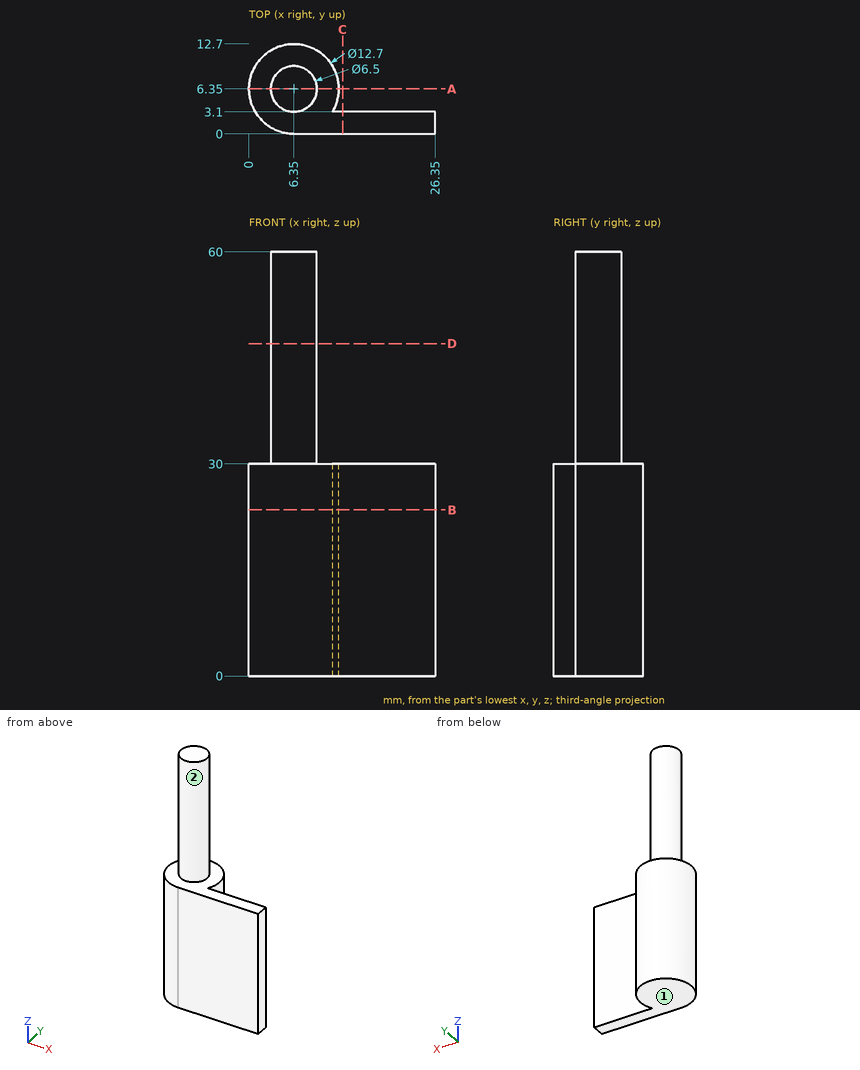
For this review, use the dimensioned drawing (mm, ordinates from the lowest corner) and the shaded views. A direction names the side the tool comes from. Coordinates: 2 decimals unless noted, no trailing zeros. Write each loop counter-clockwise with the first axis right and the second up, starting at its lowest first coordinate (ties: lowest second). Pieces come first, ordered by that corner, then holes. Notation, with made-up numbers: (-39.5, -20) - (-32.5, -20) arc R23 ccw to (-32.5, 12) - close; hole circle Ø9 at (87, -31). An arc over 180 degrees is marked (long way). Answer in a Markdown table with one row per item. Add a question column.
Q1. Clearance check with flat-ended pins moving along their axes: pin 1 (3 mm diameter, centred on y = 2.5, z = 11, fed in from -X); pin 2 (5 mm diameter, centred on x = 6.5, z = 51.5, fed in from +Y); pin 3 (2 mm diameter, centred on x = 5, z = 32.5, fed in from -Y). State where each tip first meets the part, or that it passes through.
Q2. To check wall thickness, follow line 1 along Z through (x, y) = (2, 5); line 2 along X through (y, z) = (6.75, 19.5); line 3 along Y through (x, z) = (18.25, 5.5). State the ranges of each line that lie inside material, in increasing order. Write a range as from..to.
Q3. Consider section D-D on z = 47. Give the boundary of the cut face in (x, y), then the cut area to 3 significant figures.
Q4. For the marked faces 1 and 2, list the 3-axis set-ups (+Z, -Z, +X, -X, +Y, -Y) from which the entire face can be reached by the end or side of a thin tool; tool diameter is ignored.
Q5. Consider section B-B on z = 23.5. Give the boundary of the cut face in (x, y).
Q6. Consider section C-C on x = 13.25. Give the boundary of the cut face in (y, z), then the cut area to 3 significant figures.
Q7. Consider section A-A on y = 6.35. Give the boundary of the cut face in (x, z), then the cut area to 3 significant figures.
Answers below:
| question | item | result |
|---|---|---|
| 1 | pin 1 | x = 0.45 |
| 1 | pin 2 | y = 9.6 |
| 1 | pin 3 | y = 3.12 |
| 2 | line 1 | 0..30 |
| 2 | line 2 | 0.01..12.69 |
| 2 | line 3 | 0..3.1 |
| 3 | outline | circle Ø6.5 at (6.35, 6.35) |
| 3 | area | 33.2 mm² |
| 4 | face 1 | -Z, +X, -X, +Y, -Y |
| 4 | face 2 | +Z |
| 5 | outline | (6.35, 0) - (26.35, 0) - (26.35, 3.1) - (11.81, 3.1) arc R6.35 ccw (long way) to start |
| 6 | outline | (0, 0) - (3.1, 0) - (3.1, 30) - (0, 30) - close |
| 6 | area | 93.0 mm² |
| 7 | outline | (0, 0) - (12.7, 0) - (12.7, 30) - (9.6, 30) - (9.6, 60) - (3.1, 60) - (3.1, 30) - (0, 30) - close |
| 7 | area | 576 mm² |
